```python
from build123d import *

# Parameters (mm, degrees)
F0_R     = 1.778
F1_DEPTH = 2.286
F2_W     = 6.35
F2_H     = 6.35
F3_DEPTH = 29.464
F4_R     = 1.778
F5_DEPTH = 7.62


with BuildPart() as f1:
    # F0 (on Front) → F1 (new body)
    with BuildSketch(Plane.XZ):
        Polygon((0, 6.35), (0, 0), (23.887912, 0), (30.48, 0), (30.48, 33.274), (0, 33.274), (0, 26.924), (24.104372, 26.924), (23.938964, 6.35), align=None)
        with Locations((27.305, 3.175)):
            Circle(F0_R, mode=Mode.SUBTRACT)
        with Locations((27.305, 30.099)):
            Circle(F0_R, mode=Mode.SUBTRACT)
    extrude(amount=F1_DEPTH)

    # F2 (on face) → F3 (join)
    with BuildSketch(Plane.XZ.offset(2.286)):
        with Locations((3.175, 30.099)):
            Rectangle(F2_W, F2_H)
        with Locations((3.175, 3.175)):
            Rectangle(F2_W, F2_H)
    extrude(amount=F3_DEPTH)

    # F4 (on face) → F5 (cut)
    with BuildSketch(Plane.XZ.offset(31.75)):
        with Locations((3.175, 30.099)):
            Circle(F4_R)
        with Locations((3.175, 3.175)):
            Circle(F4_R)
    extrude(amount=-F5_DEPTH, mode=Mode.SUBTRACT)


solid = f1.part
```
The model under review builds one solid part; all positions refer to its coordinate system, in mm. A direction names the side the tool comes from. Give positions to 0.01 mm unless a question says otherwise; leave off trailing zeros. Write each loop counter-clockwise with the first axis right and the second up, starting at its lowest first coordinate (ties: lowest second). Pieces come first, ordered by that corner, then holes. Notation, with made-up numbers: (32.5, 72) -> (36.5, 72) arc R34 ccw to (36.5, 109) -> close; hole circle Ø11 at (-13.75, 24). An arc over 180 degrees is marked (long way). Answer in a Markdown table with one row per item.
1) Add section D-D on z = 26. State the section outline as (x, y) points, plus the area to 3 significant figures.
Worked answers:
| item | result |
|---|---|
| outline | (24.1, -2.29) -> (30.48, -2.29) -> (30.48, 0) -> (24.1, 0) -> close |
| area | 14.6 mm² |
2) Mouldability with a two-part tool opening along X and no side actions: class faces 6 (the flat face through (30.48, -1, 16)), 7 (the flat face through (5, -12, 26.924)), 8 (the flat face through (0, -16, 30)), 9 (the flat face through (3, -24.13, 3)) as +X half, -X half, draft (parallel to the pull), parting line (faces both ways), or undercut.
Worked answers:
| item | result |
|---|---|
| face 6 | +X half |
| face 7 | draft |
| face 8 | -X half |
| face 9 | undercut |
3) Tool access review of faces 1 (the cylindrical face through (3.995, -27.993, 28.522)), 2 (the flat face through (6, -13, 33.274)), 3 (the flat face through (6.35, -17, 3)), 4 (the flat face through (6, -13, 0)), 5 (the flat face through (6, -12, 6.35)): name each direction out of +Z, -Z, +X, -X, +Y, -Y from which nothing blocks a thin tool from reaching the whole face with its end or side.
Worked answers:
| item | result |
|---|---|
| face 1 | -Y |
| face 2 | +Z, +X, -X, +Y, -Y |
| face 3 | +Z, -Z, +X, -Y |
| face 4 | -Z, +X, -X, +Y, -Y |
| face 5 | -X, +Y, -Y |
4) For L1, parallel to Z at x = 5, y = -19; L2, parallel to Y at x = 25, z = 24; L3, parallel to X at y = -5, z = 30, list the stretches that pass through material, from the lowest coordinate up. Write a range as [from, to].
Worked answers:
| item | result |
|---|---|
| L1 | [0, 6.35], [26.92, 33.27] |
| L2 | [-2.29, 0] |
| L3 | [0, 6.35] |
5) Clearance check with flat-ended pins moving along their axes: P1, Ø12, axis at x = 16, z = 16.5, coming from the -Y side; P2, Ø5, axis at y = -20, z = 29.5, coming from the +X side; P3, Ø12, axis at x = 23, z = 16, coming from the -Y side; P4, Ø4, axis at x = 3, z = 3, coming from the -Y side. State where each tip first meets the part, or that it passes through.
Worked answers:
| item | result |
|---|---|
| P1 | through |
| P2 | x = 6.35 |
| P3 | y = -2.29 |
| P4 | y = -31.75 |
6) Add section A-A on y = -7. State the section outline as (x, z) points, plus the area to 3 significant figures.
Worked answers:
| item | result |
|---|---|
| outline | (0, 0) -> (6.35, 0) -> (6.35, 6.35) -> (0, 6.35) -> close; (0, 26.92) -> (6.35, 26.92) -> (6.35, 33.27) -> (0, 33.27) -> close |
| area | 80.6 mm² |
7) Add section B-B on x = 19.5. State the section outline as (y, z) points.
Worked answers:
| item | result |
|---|---|
| outline | (-2.29, 0) -> (0, 0) -> (0, 6.35) -> (-2.29, 6.35) -> close; (-2.29, 26.92) -> (0, 26.92) -> (0, 33.27) -> (-2.29, 33.27) -> close |
8) Add section C-C on y = -25.5. State the section outline as (x, z) points (3 decimals), plus the area to 3 significant figures.
Worked answers:
| item | result |
|---|---|
| outline | (0, 0) -> (6.35, 0) -> (6.35, 6.35) -> (0, 6.35) -> close; (0, 26.924) -> (6.35, 26.924) -> (6.35, 33.274) -> (0, 33.274) -> close; hole circle Ø3.556 at (3.175, 3.175); hole circle Ø3.556 at (3.175, 30.099) |
| area | 60.8 mm² |
